Autodesk Inventor part; units mm, degrees
ref_plane "YZ Plane" through (0, 0, 0) normal (1, 0, 0) x (0, 1, 0)
ref_plane "XZ Plane" through (0, 0, 0) normal (0, 1, 0) x (-1, 0, 0)
ref_plane "XY Plane" through (0, 0, 0) normal (0, 0, 1) x (1, 0, 0)
sketch "Sketch1" plane through (0, 0, 0) normal (0, 1, 0) x (-1, 0, 0)
  line L0 (30, 50) -> (-30, 50)
  line L1 (-30, 50) -> (-30, -50)
  line L2 (-30, -50) -> (30, -50)
  line L3 (30, -50) -> (30, 50)
  line L4 (30, 50) -> (-30, -50) construction
  line L5 (-30, 50) -> (30, -50) construction
  point P0 (0, 0)
  dimension "d0" = 60
  dimension "d1" = 100
extrude "Extrusion1" add sketch "Sketch1" along normal blind 5
sketch "Sketch2" plane through (0, 5, 0) normal (0, 1, 0) x (1, 0, 0)
  circle A0 centre (15.5, -45) radius 1.25
  circle A1 centre (15.5, -32.3) radius 1.25
  line L0 (-30, -50) -> (30, -50)
  line L1 (30, -50) -> (30, 50)
  circle A2 centre (-15.5, -45) radius 1.25
  line L2 (-30, 50) -> (-30, -50)
  circle A3 centre (-15.5, -32.3) radius 1.25
  point P0 (0, 0)
  dimension "d4" = 2.5
  dimension "d5" = 2.5
  dimension "d6" = 12.7
  dimension "d7" = 5
  dimension "d8" = 14.5
  dimension "d9" = 14.5
  dimension "d10" = 2.5
  dimension "d11" = 14.5
  dimension "d12" = 2.5
extrude "Extrusion2" cut sketch "Sketch2" against normal up to next
sketch "Sketch3" plane through (0, 5, 0) normal (0, 1, 0) x (1, 0, 0)
  circle A0 centre (-17.3, 37.3) radius 4
  line L0 (30, 50) -> (-30, 50)
  line L1 (-30, 50) -> (-30, -50)
  circle A1 centre (17.3, 37.3) radius 4
  line L2 (30, -50) -> (30, 50)
  point P0 (0, 0)
  dimension "d15" = 8
  dimension "d16" = 12.7
  dimension "d17" = 12.7
  dimension "d18" = 8
  dimension "d19" = 12.7
extrude "Extrusion3" cut sketch "Sketch3" against normal up to next
fillet "Fillet1" radius 5 2 edges at (30, 2.5, 50) (-30, 2.5, 50)
properties part number "3way_final_valve_mount"
For this review, take the finished solid that the model builds, in its own axes (mm). Round coordinates to 2 decimals unless told otherwise and drop trailing zeros. Write each loop counter-clockwise with the first axis right and the second up, starting at its lowest first coordinate (ties: lowest second). Pieces come first, ordered by that corner, then holes.
1) Take a section at A-A on z = -35.5. Give the boundary of the cut face in (x, y), then the cut area to 3 significant figures.
Answer below:
outline: (-30, 0) - (-20.87, 0) - (-20.87, 5) - (-30, 5) - close; (-13.73, 0) - (13.73, 0) - (13.73, 5) - (-13.73, 5) - close; (20.87, 0) - (30, 0) - (30, 5) - (20.87, 5) - close
area: 229 mm2
2) Mouldability with a two-part tool opening along Z and no side actions: class faces 1 (the face through (15.34, 2.54, 43.76)), 2 (the face through (-15.66, 2.54, 43.76)), 3 (the face through (0, 5, 1)), 4 (the face through (28, 3, 49)) as +Z half, -Z half, draft (parallel to the pull), parting line (faces both ways), or undercut.
Answer below:
face 1: undercut
face 2: undercut
face 3: draft
face 4: +Z half
3) Take a section at C-C on x = -15.5. Give the boundary of the cut face in (y, z), then the cut area to 3 significant figures.
Answer below:
outline: (0, -50) - (5, -50) - (5, -40.87) - (0, -40.87) - close; (0, -33.73) - (5, -33.73) - (5, 31.05) - (0, 31.05) - close; (0, 33.55) - (5, 33.55) - (5, 43.75) - (0, 43.75) - close; (0, 46.25) - (5, 46.25) - (5, 50) - (0, 50) - close
area: 439 mm2
4) For line 1 along X through (y, z) = (1.9, 32.3); line 2 along X through (y, z) = (3.6, -37.3); line 3 along Z through (x, y) = (-15.5, 2.95), list the stretches that pass through material, from the lowest coordinate up.
Answer below:
line 1: x = -30 to -16.75, -14.25 to 14.25, 16.75 to 30
line 2: x = -30 to -21.3, -13.3 to 13.3, 21.3 to 30
line 3: z = -50 to -40.87, -33.73 to 31.05, 33.55 to 43.75, 46.25 to 50
5) Insertion check: pin 1 Ø4 at (x, z) = (13, 7) entering from -Y. The pin has a flat end and moves straight along its axis. Give the tip position at first contact, or say it passes through.
Answer below:
pin 1: stops at y = 0
6) Take a section at B-B on y = 2.95. Give the boundary of the cut face in (x, z).
Answer below:
outline: (-30, -50) - (30, -50) - (30, 45) arc R5 ccw to (25, 50) - (-25, 50) arc R5 ccw to (-30, 45) - close; hole circle Ø8 at (-17.3, -37.3); hole circle Ø2.5 at (-15.5, 32.3); hole circle Ø2.5 at (-15.5, 45); hole circle Ø8 at (17.3, -37.3); hole circle Ø2.5 at (15.5, 32.3); hole circle Ø2.5 at (15.5, 45)
